Can you work these out from the model? Positions are in its coordinate system, mm. A direction names the side the tool comes from. Coordinates: 2 decimals unless noted, no trailing zeros. Order: outer loops, then holes, each group sorted by start corner. A loop starts at its lowest first (then second) coordinate and runs counter-clockwise, first axis right, second up. Notation, with made-up numbers: (40, -3.5) - (92, -3.5) arc R10 cw to (92, 3.5) - close; hole circle Ø6 at (25, 36.25). An arc over 180 degrees is marked (long way). Return JSON: item names as keys, results as strings. Group by question number.
1) If I drill on line 1 along X through (y, z) = (3.7, -4.25); line 2 along X through (y, z) = (1.1, -5.5); line 3 along Y through (x, z) = (1.5, -4.25), over which ranges is the centre line in solid material (lowest first)?
2) For pin 1 Ø0.5 at (x, z) = (5, -4.5) entering from +Y, with a flat end and sliding along its axis, tell me the tip position at first contact or that it passes through.
3) Imagine slicing it at C-C (x = 5). Write out the boundary of the cut face in (y, z), and give its area (3 significant figures).
4) Imagine slicing it at A-A (y = 4.2). Write out the boundary of the cut face in (x, z), and give its area (3 significant figures).
5) If we mould it in two halves opening along X, with no side actions, what happens to faces 1 (the face through (3, 0, -4)), 2 (the face through (0.695, 2.971, -4.19)), 3 (the face through (0, 2, -4))? For each: pulls with the +X half, pulls with the -X half, needs draft (parallel to the pull), parting line crosses it, or undercut.
6) Imagine slicing it at B-B (y = 3.4). Write out the boundary of the cut face in (x, z).
7) Which directions (+Z, -Z, +X, -X, +Y, -Y) give clear straight access to the entire face, cutting with the end or side of a thin tool? Please do faces 4 (the face through (5.6, 2.9, -4.2)), 5 (the face through (2.4, 1.8, 0)).
```python
from build123d import *
from OCP.BRepFilletAPI import BRepFilletAPI_MakeChamfer

# Parameters (mm, degrees)
SKETCH1_W           = 6.3
SKETCH1_H           = 8.5
BOSS_EXTRUDE1_DEPTH = 4.8
SKETCH2_W           = 1
SKETCH2_H           = 8.5
CUT_EXTRUDE1_DEPTH  = 3.8
CHAMFER1_SIZE       = 3.8
CHAMFER1_SIZE_2     = 0.25
FILLET1_R           = 0.2
FILLET2_R           = 0.1


with BuildPart() as part:
    # Sketch1 → Boss-Extrude1 (new body)
    with BuildSketch(Plane(origin=(0, 0, 0), x_dir=(1, 0, 0), z_dir=(0, 1, 0))):
        with Locations((3.15, 4.25)):
            Rectangle(SKETCH1_W, SKETCH1_H)
    extrude(amount=BOSS_EXTRUDE1_DEPTH)

    # Sketch2 → Cut-Extrude1 (cut)
    with BuildSketch(Plane(origin=(0, 4.8, 0), x_dir=(1, 0, 0), z_dir=(0, 1, 0))):
        with Locations((1.325, 4.25)):
            Rectangle(SKETCH2_W, SKETCH2_H)
        with Locations((3.15, 4.25)):
            Rectangle(SKETCH2_W, SKETCH2_H)
        with Locations((4.975, 4.25)):
            Rectangle(SKETCH2_W, SKETCH2_H)
    extrude(amount=-CUT_EXTRUDE1_DEPTH, mode=Mode.SUBTRACT)

    # Chamfer1
    chamfer1_edges_1 = [part.edges().sort_by_distance(p)[0] for p in [
        (0.825, 4.8, -4.25),
    ]]
    chamfer1_side_1 = [part.faces().sort_by_distance(p)[0] for p in [
        (0.825, 4.795, -4.25),
    ]]
    chamfer1_edges_2 = [part.edges().sort_by_distance(p)[0] for p in [
        (5.475, 4.8, -4.25),
    ]]
    chamfer1_side_2 = [part.faces().sort_by_distance(p)[0] for p in [
        (5.48, 4.8, -4.25),
    ]]
    chamfer1_edges_3 = [part.edges().sort_by_distance(p)[0] for p in [
        (4.475, 4.8, -4.25),
    ]]
    chamfer1_side_3 = [part.faces().sort_by_distance(p)[0] for p in [
        (4.475, 4.795, -4.25),
    ]]
    chamfer1_edges_4 = [part.edges().sort_by_distance(p)[0] for p in [
        (3.65, 4.8, -4.25),
    ]]
    chamfer1_side_4 = [part.faces().sort_by_distance(p)[0] for p in [
        (3.655, 4.8, -4.25),
    ]]
    chamfer1_edges_5 = [part.edges().sort_by_distance(p)[0] for p in [
        (2.65, 4.8, -4.25),
    ]]
    chamfer1_side_5 = [part.faces().sort_by_distance(p)[0] for p in [
        (2.65, 4.795, -4.25),
    ]]
    chamfer1_edges_6 = [part.edges().sort_by_distance(p)[0] for p in [
        (1.825, 4.8, -4.25),
    ]]
    chamfer1_side_6 = [part.faces().sort_by_distance(p)[0] for p in [
        (1.83, 4.8, -4.25),
    ]]
    chamfer1 = BRepFilletAPI_MakeChamfer(part.part.solid().wrapped)
    for e in chamfer1_edges_1:
        chamfer1.Add(CHAMFER1_SIZE - 0.0001, CHAMFER1_SIZE_2 - 0.0001, e.wrapped, chamfer1_side_1[0].wrapped)
    for e in chamfer1_edges_2:
        chamfer1.Add(CHAMFER1_SIZE_2 - 0.0001, CHAMFER1_SIZE - 0.0001, e.wrapped, chamfer1_side_2[0].wrapped)
    for e in chamfer1_edges_3:
        chamfer1.Add(CHAMFER1_SIZE - 0.0001, CHAMFER1_SIZE_2 - 0.0001, e.wrapped, chamfer1_side_3[0].wrapped)
    for e in chamfer1_edges_4:
        chamfer1.Add(CHAMFER1_SIZE_2 - 0.0001, CHAMFER1_SIZE - 0.0001, e.wrapped, chamfer1_side_4[0].wrapped)
    for e in chamfer1_edges_5:
        chamfer1.Add(CHAMFER1_SIZE - 0.0001, CHAMFER1_SIZE_2 - 0.0001, e.wrapped, chamfer1_side_5[0].wrapped)
    for e in chamfer1_edges_6:
        chamfer1.Add(CHAMFER1_SIZE_2 - 0.0001, CHAMFER1_SIZE - 0.0001, e.wrapped, chamfer1_side_6[0].wrapped)
    add(Compound.cast(chamfer1.Shape()), mode=Mode.REPLACE)  # a hair under: the kernel refuses the full size

    # Fillet1
    fillet1_edges = [part.edges().sort_by_distance(p)[0] for p in [
        (0.825, 1, -4.25),
        (1.825, 1, -4.25),
        (2.65, 1, -4.25),
        (3.65, 1, -4.25),
        (4.475, 1, -4.25),
        (5.475, 1, -4.25),
    ]]
    fillet(fillet1_edges, radius=FILLET1_R)

    # Fillet2
    fillet2_edges = [part.edges().sort_by_distance(p)[0] for p in [
        (6.3, 4.8, -4.25),
        (0, 4.8, -4.25),
        (5.7249, 4.8, -4.25),
        (3.8999, 4.8, -4.25),
        (4.2251, 4.8, -4.25),
        (2.0749, 4.8, -4.25),
        (2.4001, 4.8, -4.25),
        (0.5751, 4.8, -4.25),
    ]]
    fillet(fillet2_edges, radius=FILLET2_R)


solid = part.part
```
Calculated:
{
 "1": {"line 1": "0 to 0.65, 2 to 2.47, 3.83 to 4.3, 5.65 to 6.3", "line 2": "0 to 0.84, 1.81 to 2.66, 3.64 to 4.49, 5.46 to 6.3", "line 3": "0 to 1"},
 "2": {"pin 1": "y = 1"},
 "3": {"outline": "(0, -8.5) - (1, -8.5) - (1, 0) - (0, 0) - close", "area": "8.50 mm2"},
 "4": {"outline": "(0, -8.5) - (0.61, -8.5) - (0.61, 0) - (0, 0) - close; (2.04, -8.5) - (2.44, -8.5) - (2.44, 0) - (2.04, 0) - close; (3.86, -8.5) - (4.26, -8.5) - (4.26, 0) - (3.86, 0) - close; (5.69, -8.5) - (6.3, -8.5) - (6.3, 0) - (5.69, 0) - close", "area": "17.3 mm2"},
 "5": {"face 1": "needs draft", "face 2": "undercut", "face 3": "pulls with the -X half"},
 "6": {"outline": "(0, -8.5) - (0.67, -8.5) - (0.67, 0) - (0, 0) - close; (1.98, -8.5) - (2.49, -8.5) - (2.49, 0) - (1.98, 0) - close; (3.81, -8.5) - (4.32, -8.5) - (4.32, 0) - (3.81, 0) - close; (5.63, -8.5) - (6.3, -8.5) - (6.3, 0) - (5.63, 0) - close"},
 "7": {"face 4": "+Z, -Z, +Y", "face 5": "+Z, +X, -X, +Y, -Y"}
}
